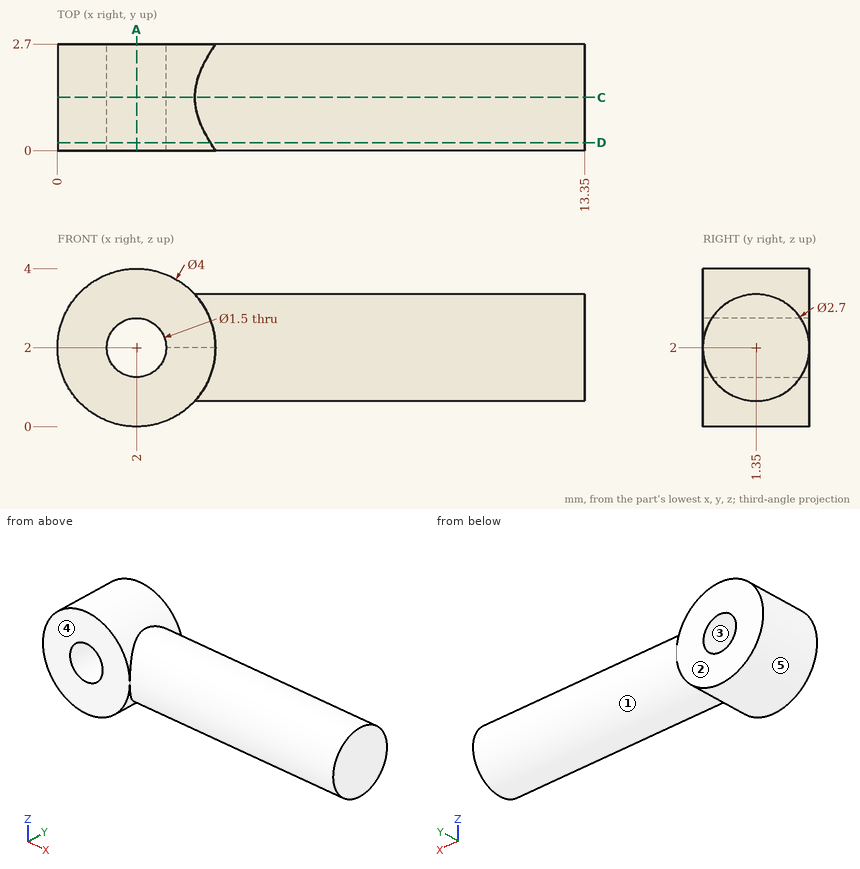
Verification items for this drawing (mm, ordinates from the low corner). A direction names the side the tool comes from. Round coordinates to 2 decimals unless told otherwise and drop trailing zeros. Order: outer loops, then holes, each group sorted by start corner. A loop starts at its lowest first (then second) coordinate and runs counter-clockwise, first axis right, second up.
1) Cross-section at A-A, the plane x = 2. Record the cut outline in (y, z).
Geometry says:
outline: (0, 0) - (2.7, 0) - (2.7, 1.25) - (0, 1.25) - close; (0, 2.75) - (2.7, 2.75) - (2.7, 4) - (0, 4) - close
2) Cross-section at D-D, the plane y = 0.2. Record the cut outline in (x, z).
Geometry says:
outline: (3.87, 1.29) - (13.35, 1.29) - (13.35, 2.71) - (3.87, 2.71) arc R2 ccw (long way) to start; hole circle Ø1.5 at (2, 2)
3) Tool access check on the marked faces 1 and 2. Record the directions out of +Z, -Z, +X, -X, +Y, -Y that give a thin tool (end or side, any length) a straight path to the whole face; none if there is none.
Geometry says:
face 1: +X
face 2: +Z, -Z, +X, -X, +Y
4) Draft check along X on the marked faces 3, 4 and 5. Enter one of: +X half, -X half, draft (parallel to the pull), parting line (faces both ways), or undercut.
Geometry says:
face 3: undercut
face 4: draft
face 5: parting line
5) Cross-section at C-C, the plane y = 1.35. Record the cut outline in (x, z), plus the area to 3 significant figures.
Geometry says:
outline: (3.48, 0.65) - (13.35, 0.65) - (13.35, 3.35) - (3.48, 3.35) arc R2 ccw (long way) to start; hole circle Ø1.5 at (2, 2)
area: 36.5 mm2
6) Material ranges on line 1 (Z direction, x = 1.5, y = 2.1); line 2 (X direction, y = 0.3, z = 2.2); line 3 (Z direction, x = 5.25, y = 1.4), recorded low to high.
Geometry says:
line 1: z = 0.06 to 1.44, 2.56 to 3.94
line 2: x = 0.01 to 1.28, 2.72 to 13.35
line 3: z = 0.65 to 3.35
7) Depth check by flat-ended pin: pin 1 (1.5 mm diameter, centred on x = 8.5, y = 1.5, fed in from -Z); pin 2 (1.2 mm diameter, centred on x = 2, z = 2, fed in from +Y). Enter the tip coordinate at first touch or a pass-through.
Geometry says:
pin 1: stops at z = 0.65
pin 2: passes through
